Input: part model. Units: mm. Frame: model coordinates. A direction names the side the tool comes from. Give positions to 0.01 mm unless a question says otherwise; leave off trailing zeros. Loops run counter-clockwise (first coordinate to the right, second up) from the corner with the lowest first, then second, coordinate; pieces in that order, holes last. Notation, with made-up numbers: (51.25, -2.75) - (101.25, -2.75) arc R9 ccw to (101.25, 8.25) - close; hole circle Ø7 at (6.5, 43). An arc over 180 degrees is marked (long way). One line per item, written item: value.
from build123d import *

# Parameters (mm, degrees)
SKETCH1_W           = 25.4
SKETCH1_H           = 25.4
BOSS_EXTRUDE1_DEPTH = 6.35
SKETCH2_W           = 25.4
SKETCH2_H           = 25.4
BOSS_EXTRUDE2_DEPTH = 6.35
FILLET1_R           = 3.175
FILLET2_R           = 2.3876
SKETCH3_R           = 3.3782
CUT_EXTRUDE1_DEPTH  = 7.35
SKETCH4_R           = 3.3782
CUT_EXTRUDE2_DEPTH  = 7.35


with BuildPart() as part:
    # Sketch1 → Boss-Extrude1 (new body)
    with BuildSketch(Plane(origin=(0, 0, 0), x_dir=(1, 0, 0), z_dir=(0, 1, 0))):
        with Locations((12.7, 12.7)):
            Rectangle(SKETCH1_W, SKETCH1_H)
    extrude(amount=BOSS_EXTRUDE1_DEPTH)

    # Sketch2 → Boss-Extrude2 (add)
    with BuildSketch(Plane(origin=(0, 0, -25.4), x_dir=(-1, 0, 0), z_dir=(0, 0, -1))):
        with Locations((-12.7, 12.7)):
            Rectangle(SKETCH2_W, SKETCH2_H)
    extrude(amount=-BOSS_EXTRUDE2_DEPTH)

    # Fillet1
    fillet1_edges = [part.edges().sort_by_distance(p)[0] for p in [
        (12.7, 6.35, -19.05),
    ]]
    fillet(fillet1_edges, radius=FILLET1_R)

    # Fillet2
    fillet2_edges = [part.edges().sort_by_distance(p)[0] for p in [
        (12.7, 25.4, -19.05),
        (12.7, 6.35, 0),
    ]]
    fillet(fillet2_edges, radius=FILLET2_R)

    # Sketch3 → Cut-Extrude1 (cut, through all)
    with BuildSketch(Plane(origin=(0, 6.35, 0), x_dir=(1, 0, 0), z_dir=(0, 1, 0))):
        with Locations((12.7, 9.1313)):
            Circle(SKETCH3_R)
        with Locations((29.80436, 9.1313)):
            Circle(SKETCH3_R)
        with Locations((46.39564, 9.1313)):
            Circle(SKETCH3_R)
        with Locations((33.500058156, 19.57038717)):
            Circle(SKETCH3_R)
    extrude(amount=-CUT_EXTRUDE1_DEPTH, mode=Mode.SUBTRACT)

    # Sketch4 → Cut-Extrude2 (cut, through all)
    with BuildSketch(Plane.XY.offset(-19.05)):
        with Locations((-37.07384, 16.2687)):
            Circle(SKETCH4_R)
        with Locations((-20.48256, 16.2687)):
            Circle(SKETCH4_R)
        with Locations((-3.89128, 16.2687)):
            Circle(SKETCH4_R)
        with Locations((12.7, 16.2687)):
            Circle(SKETCH4_R)
    extrude(amount=-CUT_EXTRUDE2_DEPTH, mode=Mode.SUBTRACT)


solid = part.part
Item 1: Section B-B, the plane y = 13.5. Output: boundary loops of the cut face in (x, z), and give its area (3 significant figures).
Verdict:
outline: (0, -25.4) - (10.76, -25.4) - (10.76, -19.05) - (0, -19.05) - close; (14.64, -25.4) - (25.4, -25.4) - (25.4, -19.05) - (14.64, -19.05) - close
area: 137 mm^2
Item 2: Section C-C, the plane z = -8.5. Output: boundary loops of the cut face in (x, y).
Verdict:
outline: (0, 0) - (9.38, 0) - (9.38, 6.35) - (0, 6.35) - close; (16.02, 0) - (25.4, 0) - (25.4, 6.35) - (16.02, 6.35) - close
Item 3: Section A-A, the plane x = 12.7. Count the separate pieces of the cut face and the enclosed holes in it, and give its area (3 significant figures).
Verdict:
separate pieces: 3
enclosed holes: 0
area: 196 mm^2
Item 4: Draft query along Z for faces 3 (the face through (13, 0, -13)), 4 (the face through (10.21, 3.219, -11.414)), 5 (the face through (12.52, 24.68, -19.73)). Return one class per face: pulls with the +Z half, pulls with the -Z half, needs draft (parallel to the pull), parting line crosses it, or undercut.
Verdict:
face 3: needs draft
face 4: undercut
face 5: pulls with the +Z half
Item 5: Material intervals for L1, parallel to Z at x = 12.7, y = 1.5; L2, parallel to Y at x = 12.7, z = -21.25; L3, parallel to Z at x = 19.25, y = 14, sorted ascending.
Verdict:
L1: z = -25.4 to -12.51, -5.75 to 0
L2: y = 0 to 12.89, 19.65 to 25.39
L3: z = -25.4 to -19.05
Item 6: Access query for faces 1 (the face through (16, 18, -19.05)), 2 (the face through (13, 25.4, -23)). Directions: +Z, -Z, +X, -X, +Y, -Y. A direction counts if a zero-diameter tool reaches every point of the face in a straight line with its end or side. Return the directions, or none.
Verdict:
face 1: +Z, +X, -X, +Y
face 2: +Z, -Z, +X, -X, +Y
Item 7: Section D-D, the plane x = 6.75. Output: boundary loops of the cut face in (y, z) (3 decimals).
Verdict:
outline: (0, -25.4) - (25.4, -25.4) - (25.4, -21.438) arc R2.388 ccw to (23.012, -19.05) - (9.525, -19.05) arc R3.175 cw to (6.35, -15.875) - (6.35, -2.388) arc R2.388 ccw to (3.962, 0) - (0, 0) - close
Item 8: Pin query (flat end, axial travel): P1, Ø11, axis at x = 12.7, y = 16.27, coming from the +Z side; P2, Ø12, axis at x = 7, z = -6.5, coming from the +Y side; P3, Ø6, axis at x = 12.7, z = -9.13, coming from the +Y side; P4, Ø2, axis at x = 18, y = 17.5, coming from the +Z side. Return the tip coordinate at first contact, or that it passes through.
Verdict:
P1: stops at z = -19.05
P2: stops at y = 6.35
P3: passes through
P4: stops at z = -19.05
